Here's how the part is built. I have some questions about the finished solid (model axes, mm). A direction names the side the tool comes from. Give positions to 0.01 mm unless a question says otherwise; leave off trailing zeros. Loops run counter-clockwise (first coordinate to the right, second up) from the corner with the lowest first, then second, coordinate; pieces in that order, holes last. Notation, with made-up numbers: (87.25, 8.5) - (104.25, 8.5) arc R9 cw to (104.25, 23.5) - close; hole circle Ø11 at (72.25, 46). An arc over 180 degrees is marked (long way). Use one line per item in the form item = value.
Autodesk Inventor part; units mm, degrees
ref_plane "YZ Plane" through (0, 0, 0) normal (1, 0, 0) x (0, 1, 0)
ref_plane "XZ Plane" through (0, 0, 0) normal (0, 1, 0) x (-1, 0, 0)
ref_plane "XY Plane" through (0, 0, 0) normal (0, 0, 1) x (1, 0, 0)
sketch "Sketch5" plane through (0, 0, 0) normal (0, 1, 0) x (-1, 0, 0)
  line L0 (9.4203, 11.6048) -> (-50.5797, 11.6048)
  line L1 (-50.5797, 11.6048) -> (-50.5797, -27.8952)
  line L2 (-50.5797, -27.8952) -> (9.4203, -27.8952)
  line L3 (9.4203, -27.8952) -> (9.4203, 11.6048)
  circle A0 centre (2.6703, 4.8548) radius 1.75
  circle A1 centre (2.6703, -21.1452) radius 1.75
  circle A2 centre (-39.3297, 8.8548) radius 1.75
  circle A3 centre (-39.3297, -25.1452) radius 1.75
  line L4 (-36.9794, -23.1452) -> (-34.9794, -23.1452)
  line L5 (-34.9794, -23.1452) -> (-34.9794, 6.8548)
  line L6 (-34.9794, 6.8548) -> (-36.9794, 6.8548)
  line L7 (-36.9794, 6.8548) -> (-36.9794, -23.1452)
  line L8 (7.9203, 6.8548) -> (5.9203, 6.8548)
  line L9 (5.9203, 6.8548) -> (5.9203, -23.1452)
  line L10 (5.9203, -23.1452) -> (7.9203, -23.1452)
  line L11 (7.9203, -23.1452) -> (7.9203, 6.8548)
  point P0 (0, 0)
  dimension "d9" = 60
  dimension "d10" = 39.5
  dimension "d11" = 3.5
  dimension "d12" = 3.5
  dimension "d13" = 3.5
  dimension "d14" = 3.5
  dimension "d16" = 6.75
  dimension "d17" = 6.75
  dimension "d18" = 6.75
  dimension "d19" = 6.75
  dimension "d20" = 11.25
  dimension "d21" = 2.75
  dimension "d22" = 11.25
  dimension "d23" = 2.75
  dimension "d24" = 2
  dimension "d25" = 2
  dimension "d26" = 30
  dimension "d27" = 4.75
  dimension "d28" = 4.75
  dimension "d29" = 2
  dimension "d30" = 30
  dimension "d31" = 1.5
  dimension "d32" = 4.75
  dimension "d33" = 4.75
extrude "Extrusion2" add sketch "Sketch5" against normal blind 1.5 contours L3 L2 L1 L0 | A0 | A1 | A2 | A3 | L7 L6 L5 L4 | L11 L10 L9 L8
extrude "Extrusion3" add sketch "Sketch5" along normal blind 6 contours A0 | A1 | A2 | A3
extrude "Extrusion4" add sketch "Sketch5" along normal blind 3.5 contours L7 L6 L5 L4 | L11 L10 L9 L8
properties part number "RFID-RC522 Holder 3.0"
(1) If I drill on probe 1 along X at (y, z) = (1.75, 5); probe 2 along X at (y, z) = (1.5, -13); probe 3 along Y at (x, z) = (2, 8), over which ranges is the centre line in solid material (lowest first)?
Geometry says:
probe_1 = -7.92 to -5.92, -4.41 to -0.93, 34.98 to 36.98
probe_2 = -7.92 to -5.92, 34.98 to 36.98
probe_3 = -1.5 to 0
(2) For P1, Ø12, axis at x = 11.5, z = -7.5, coming from the +Y side; P2, Ø0.6, axis at x = -7, y = 1.5, coming from the +Z side; P3, Ø1, axis at x = 36.5, y = 1.5, coming from the -Z side; P4, Ø4, axis at x = 25.5, y = 0.5, coming from the +Z side, each with a flat end and sliding along its axis, tell me the tip position at first contact or that it passes through.
Geometry says:
P1 = 0
P2 = 6.85
P3 = -23.15
P4 = 11.6
(3) If we section it at A-A (z = -5): List the corners of the cut face in (x, y) for me, plus the area to 3 significant figures.
Geometry says:
outline = (-9.42, -1.5) - (50.58, -1.5) - (50.58, 0) - (36.98, 0) - (36.98, 3.5) - (34.98, 3.5) - (34.98, 0) - (-5.92, 0) - (-5.92, 3.5) - (-7.92, 3.5) - (-7.92, 0) - (-9.42, 0) - close
area = 104 mm²
(4) For faces 5 (the flat face through (-7.92, 2, -8)), 6 (the cylindrical face through (-2.44, 2.96, -22.88)), 7 (the flat face through (34.979, 2, -8)), 8 (the flat face through (36.979, 2, -8)), which set-ups out of +Z, -Z, +X, -X, +Y, -Y let a thin tool reach every point of the face, with its end or its side?
Geometry says:
face_5 = +Z, -Z, -X, +Y
face_6 = +Y
face_7 = +Z, -Z, +Y
face_8 = +Z, -Z, +X, +Y
(5) If we section it at C-C (x = -2): List the corners of the cut face in (y, z) for me.
Geometry says:
outline = (-1.5, -27.9) - (0, -27.9) - (0, -22.76) - (6, -22.76) - (6, -19.53) - (0, -19.53) - (0, 3.24) - (6, 3.24) - (6, 6.47) - (0, 6.47) - (0, 11.6) - (-1.5, 11.6) - close
(6) If we section it at D-D (x = 21): List the corners of the cut face in (y, z) for me, plus the area to 4 significant figures.
Geometry says:
outline = (-1.5, -27.9) - (0, -27.9) - (0, 11.6) - (-1.5, 11.6) - close
area = 59.25 mm²
(7) If we section it at B-B (y = 1): List the corners of the cut face in (x, z) for me.
Geometry says:
outline = (-7.92, -23.15) - (-5.92, -23.15) - (-5.92, 6.85) - (-7.92, 6.85) - close; circle Ø3.5 at (-2.67, -21.15); circle Ø3.5 at (-2.67, 4.85); (34.98, -23.15) - (36.98, -23.15) - (36.98, 6.85) - (34.98, 6.85) - close; circle Ø3.5 at (39.33, -25.15); circle Ø3.5 at (39.33, 8.85)
(8) Thinking about a two-plate mould opening in Z: for faces 1 (the cylindrical face through (37.66, 2.96, -25.67)), 2 (the flat face through (-5.92, 2, -8)), 3 (the flat face through (-7, 2, 6.855)), 4 (the cylindrical face through (37.713, 2.958, 9.525)), which applies, pulls with the +Z half, pulls with the -Z half, needs draft (parallel to the pull), parting line crosses it, or undercut?
Geometry says:
face_1 = undercut
face_2 = needs draft
face_3 = pulls with the +Z half
face_4 = undercut
